```python
from build123d import *

# Parameters (mm, degrees)
SKETCH1_W           = 120
SKETCH1_H           = 150
BOSS_EXTRUDE1_DEPTH = 40
FILLET2_R           = 5
SKETCH2_W           = 110
SKETCH2_H           = 140
CUT_EXTRUDE1_DEPTH  = 30


with BuildPart() as part:
    # Sketch1 → Boss-Extrude1 (new body)
    with BuildSketch(Plane.XY):
        with Locations((-27.929641074, 46.164250059)):
            Rectangle(SKETCH1_W, SKETCH1_H)
    extrude(amount=BOSS_EXTRUDE1_DEPTH)

    # Fillet2
    fillet2_edges = [part.edges().sort_by_distance(p)[0] for p in [
        (-87.929641074, 46.164250059, 40),
        (-27.929641074, -28.835749941, 40),
        (32.070358926, 46.164250059, 40),
        (-27.929641074, -28.835749941, 0),
        (-87.929641074, 46.164250059, 0),
        (-27.929641074, 121.164250059, 0),
        (32.070358926, 46.164250059, 0),
        (-27.929641074, 121.164250059, 40),
        (32.070358926, -28.835749941, 20),
        (-87.929641074, -28.835749941, 20),
        (-87.929641074, 121.164250059, 20),
        (32.070358926, 121.164250059, 20),
    ]]
    fillet(fillet2_edges, radius=FILLET2_R)

    # Sketch2 → Cut-Extrude1 (cut)
    with BuildSketch(Plane.XY.offset(40)):
        with Locations((-27.929641074, 46.164250059)):
            Rectangle(SKETCH2_W, SKETCH2_H)
    extrude(amount=-CUT_EXTRUDE1_DEPTH, mode=Mode.SUBTRACT)


solid = part.part
```
The model under review builds one solid part; all positions refer to its coordinate system, in mm. A direction names the side the tool comes from. Round coordinates to 2 decimals unless told otherwise and drop trailing zeros. Write each loop counter-clockwise with the first axis right and the second up, starting at its lowest first coordinate (ties: lowest second). Pieces come first, ordered by that corner, then holes. Notation, with made-up numbers: (30.25, -38) - (77.25, -38) arc R35 cw to (77.25, 1) - close; hole circle Ø5 at (21.25, 36.5). An arc over 180 degrees is marked (long way). Use one line per item in the form item = value.
Q1. Insertion check: pin 1 Ø2 at (x, y) = (-10.5, 4.5) entering from +Z. The pin has a flat end and moves straight along its axis. Give the tip position at first contact, or say it passes through.
Answer key:
pin_1 = 10
Q2. For line 1 (Y direction, x = -44, z = 34); line 2 (X direction, y = 105, z = 28); line 3 (Z direction, x = -46.5, y = 95.5), list the stretches that pass through material, from the lowest coordinate up. Write a range as [from, to].
Answer key:
line_1 = [-28.84, -23.84], [116.16, 121.16]
line_2 = [-87.93, -82.93], [27.07, 32.07]
line_3 = [0, 10]
Q3. Tool access review of faces 4 (the flat face through (-82.93, 45, 25)), 5 (the cylindrical face through (30.567, -27.41, 20.21)): name each direction out of +Z, -Z, +X, -X, +Y, -Y from which nothing blocks a thin tool from reaching the whole face with its end or side.
Answer key:
face_4 = +Z
face_5 = +Z, -Z, +X, -Y
Q4. Consider section B-B (x = -56). State the section outline as (y, z) points, and give its area (3 significant figures).
Answer key:
outline = (-28.84, 5) arc R5 ccw to (-23.84, 0) - (116.16, 0) arc R5 ccw to (121.16, 5) - (121.16, 35) arc R5 ccw to (116.16, 40) - (116.16, 10) - (-23.84, 10) - (-23.84, 40) arc R5 ccw to (-28.84, 35) - close
area = 1,780 mm2
Q5. Consider section A-A (z = 15.5). State the section outline as (x, y) points.
Answer key:
outline = (-87.93, -23.84) arc R5 ccw to (-82.93, -28.84) - (27.07, -28.84) arc R5 ccw to (32.07, -23.84) - (32.07, 116.16) arc R5 ccw to (27.07, 121.16) - (-82.93, 121.16) arc R5 ccw to (-87.93, 116.16) - close; hole (-82.93, -23.84) - (27.07, -23.84) - (27.07, 116.16) - (-82.93, 116.16) - close
Q6. Consider section C-C (y = 16). State the section outline as (x, z) points, and give its area (3 significant figures).
Answer key:
outline = (-87.93, 5) arc R5 ccw to (-82.93, 0) - (27.07, 0) arc R5 ccw to (32.07, 5) - (32.07, 35) arc R5 ccw to (27.07, 40) - (27.07, 10) - (-82.93, 10) - (-82.93, 40) arc R5 ccw to (-87.93, 35) - close
area = 1,480 mm2
Q7. Draft analysis for pull direction Y (two halves, no side actions). For faces 1 (the flat face through (-29, -23.836, 25)), 2 (the cylindrical face through (-86.5, 47.1, 38.5)), 3 (the cylindrical face through (-27.16, -27.41, 1.504)), state which applies: +Y half, -Y half, draft (parallel to the pull), parting line (faces both ways), or undercut.
Answer key:
face_1 = undercut
face_2 = draft
face_3 = -Y half
